```python
from build123d import *

# Parameters (mm, degrees)
R_P_TITION_CIRCULAIRE1_COUNT = 4


with BuildPart() as part:
    # Esquisse1 → Base-Révolution (revolve)
    with BuildSketch(Plane.XY):
        with BuildLine():
            Line((-8, 2.5), (8, 2.5))
            ThreePointArc((8, 2.5), (8.499595763, 1.294111664), (8.67, 0))
            Line((8.67, 0), (-8.67, 0))
            ThreePointArc((-8.67, 0), (-8.499595763, 1.294111664), (-8, 2.5))
        make_face()
    revolve(axis=Axis((0, 0, 0), (-1, 0, 0)))

    # Esquisse2 → Enlever de la matière-Révolution1 (revolve, cut)
    with BuildSketch(Plane(origin=(0, 2.5, 0), x_dir=(-1, 0, 0), z_dir=(0, 1, 0))):
        with BuildLine():
            Line((1.333333333, 0), (-1.333333333, 0))
            ThreePointArc((-1.333333333, 0), (-0.687386859, 0.249968429), (0, 0.335))
            ThreePointArc((0, 0.335), (0.687386859, 0.249968429), (1.333333333, 0))
        make_face()
    enlever_de_la_mati_re_r_volution1 = revolve(axis=Axis((0, 2.5, 0), (1, 0, 0)), mode=Mode.SUBTRACT)

    # Répétition circulaire1: Enlever de la matière-Révolution1 ×4 about axis
    r_p_tition_circulaire1_axis = Axis((50, 0, 0), (-1, 0, 0))
    for i in range(1, R_P_TITION_CIRCULAIRE1_COUNT):
        add(enlever_de_la_mati_re_r_volution1.rotate(r_p_tition_circulaire1_axis, i * 360 / R_P_TITION_CIRCULAIRE1_COUNT), mode=Mode.SUBTRACT)


solid = part.part
```
Geometry: final body of the model. Coordinates: model frame, mm. Coordinates: 2 decimals unless noted, no trailing zeros. Order: outer loops, then holes, each group sorted by start corner. A loop starts at its lowest first (then second) coordinate and runs counter-clockwise, first axis right, second up. Notation, with made-up numbers: (46.25, 11) - (61.25, 11) arc R6 ccw to (61.25, 19) - close; hole circle Ø9 at (50.5, 65.25). An arc over 180 degrees is marked (long way). Return JSON: item names as keys, results as strings. Group by question number.
1. Cut plane A-A (x = -5). Output: boundary loops of the cut face in (y, z).
2. Pin query (flat end, axial travel): pin 1 (1.5 mm diameter, centred on y = -0.5, z = 1.5, fed in from +X); pin 2 (1 mm diameter, centred on x = -6, y = -1.5, fed in from -Z). Return the tip coordinate at first contact, or that it passes through.
3. Cut plane C-C (y = -0.9). Output: boundary loops of the cut face in (x, z) (1 decimal).
4. Cut plane B-B (z = -1.9). Output: boundary loops of the cut face in (x, y), plus the area to 3 significant figures.
5. Material intervals for line 1 along Z through (x, y) = (-5, -0.15); line 2 along Z through (x, y) = (-5, -1.3); line 3 along X through (y, z) = (0.2, -0.9), sorted ascending. Write a range as [from, to].
Resolved:
{
 "1": {"outline": "circle Ø5 at (0, 0)"},
 "2": {"pin 1": "stops at x = 8.6", "pin 2": "stops at z = -2.29"},
 "3": {"outline": "(-8, -2.3) - (8, -2.3) arc R4.9 ccw to (8, 2.3) - (-8, 2.3) arc R4.9 ccw to start"},
 "4": {"outline": "(-8, -1.62) - (8, -1.62) arc R4.62 ccw to (8, 1.62) - (-8, 1.62) arc R4.62 ccw to start", "area": "53.3 mm²"},
 "5": {"line 1": "z = [-2.5, 2.5]", "line 2": "z = [-2.14, 2.14]", "line 3": "x = [-8.58, 8.58]"}
}
